Geometry: final body of the model. Coordinates: model frame, mm. A direction names the side the tool comes from. Give positions to 0.01 mm unless a question says otherwise; leave off trailing zeros. Write each loop counter-clockwise with the first axis right and the second up, starting at its lowest first coordinate (ties: lowest second). Pieces come first, ordered by that corner, then holes. Notation, with made-up numbers: (42.25, 59) - (50.25, 59) arc R6 ccw to (50.25, 68) - close; hole circle Ø8 at (48.5, 42.25). An arc over 180 degrees is marked (long way). One line per question, with ' | ' between items. Start each with the question number.
```python
from build123d import *

# Parameters (mm, degrees)
EXTRUDE_2_DEPTH          = 5
FILLET_3_R               = 1
SKETCH_3_R               = 13
SKETCH_3_R_2             = 1.6
CUT_EXTRUDE_5_DEPTH      = 5
CUT_EXTRUDE_6_DEPTH      = 54.322134241
CUT_EXTRUDE_6_DEPTH_BACK = 54.322134241
SKETCH_4_R               = 1.525
CUT_EXTRUDE_7_DEPTH      = 10
FILLET_4_R               = 1.5


with BuildPart() as part:
    # 草圖2 → 填料-伸長2 (new body)
    with BuildSketch(Plane.XY):
        with BuildLine():
            Line((-26.5, 46), (26.5, 46))
            Line((26.5, 46), (26.5, 36))
            Line((26.5, 36), (23, 0))
            ThreePointArc((23, 0), (0, -23), (-23, 0))
            Line((-23, 0), (-26.5, 36))
            Line((-26.5, 36), (-26.5, 46))
        make_face()
    extrude(amount=EXTRUDE_2_DEPTH)

    # 圓角3
    # the kernel refuses this fillet: 1 mm, written as the material it takes off along each edge
    with BuildSketch(Plane(origin=(-26.5, 46, -2.5), x_dir=(0, -1, 0), z_dir=(0, 0, 1)), Plane(origin=(26.5, 46, -2.5), x_dir=(-1, 0, 0), z_dir=(0, 0, 1))) as fillet_3_piece_1:
        with BuildLine():
            CenterArc((FILLET_3_R, FILLET_3_R), FILLET_3_R, 180, 90)
            Line((0, FILLET_3_R), (0, 0))
            Line((0, 0), (FILLET_3_R, 0))
        make_face()
    extrude(amount=10, mode=Mode.SUBTRACT)
    with BuildSketch(Plane(origin=(26.5, 36, -0.121241952), x_dir=(0, 1, 0), z_dir=(0, 0, 1)), Plane(origin=(-26.5, 36, -0.121241952), x_dir=(0.0967659740606196, -0.9953071617667079, 0), z_dir=(0, 0, 1))) as fillet_3_piece_2:
        with BuildLine():
            CenterArc((FILLET_3_R * 0.0484967808039, FILLET_3_R), FILLET_3_R, 264.447028967, 5.552971033)
            Line((-FILLET_3_R * 0.0482691932568, FILLET_3_R * 0.0046928382333), (0, 0))
            Line((0, 0), (FILLET_3_R * 0.0484967808039, 0))
        make_face()
    extrude(amount=5.242483904, mode=Mode.SUBTRACT)

    # 草圖3 → 除料-伸長5 (cut)
    with BuildSketch(Plane.XY):
        Circle(SKETCH_3_R)
        with Locations((18.009998301, 0)):
            Circle(SKETCH_3_R_2)
        with Locations((0, -18.009998301)):
            Circle(SKETCH_3_R_2)
        with Locations((-18.009998301, 0)):
            Circle(SKETCH_3_R_2)
        with Locations((0, 18.009998301)):
            Circle(SKETCH_3_R_2)
        with Locations((11.999602077, 11.999602077)):
            Circle(SKETCH_3_R_2)
        with Locations((11.999602077, -11.999602077)):
            Circle(SKETCH_3_R_2)
        with Locations((-11.999602077, -11.999602077)):
            Circle(SKETCH_3_R_2)
        with Locations((-11.999602077, 11.999602077)):
            Circle(SKETCH_3_R_2)
    extrude(amount=CUT_EXTRUDE_5_DEPTH, mode=Mode.SUBTRACT)

    # 草圖4 → 除料-伸長6 (cut, two sides: drawn at the far end of the back side and taken through both)
    with BuildSketch(Plane.XY.offset(-CUT_EXTRUDE_6_DEPTH_BACK)):
        with Locations((21, 41)):
            Circle(SKETCH_4_R)
        with Locations((7, 41)):
            Circle(SKETCH_4_R)
        with Locations((-7, 41)):
            Circle(SKETCH_4_R)
        with Locations((-21, 41)):
            Circle(SKETCH_4_R)
    extrude(amount=CUT_EXTRUDE_6_DEPTH + CUT_EXTRUDE_6_DEPTH_BACK, mode=Mode.SUBTRACT)

    # 草圖5 → 除料-伸長7 (cut)
    with BuildSketch(Plane.XY.offset(5)):
        Polygon((-21.5, 35), (-6.5, 35), (-20.2, 21), align=None)
        Polygon((11.3, 22.7), (-11.3, 22.7), (0, 34.95), align=None)
        Polygon((6.5, 35), (20.2, 21), (21.5, 35), align=None)
    extrude(amount=-CUT_EXTRUDE_7_DEPTH, mode=Mode.SUBTRACT)

    # 圓角4
    fillet_4_edges = [part.edges().sort_by_distance(p)[0] for p in [
        (6.5, 35, 2.5),
        (21.5, 35, 2.5),
        (20.2, 21, 2.5),
        (-11.3, 22.7, 2.5),
        (0, 34.95, 2.5),
        (11.3, 22.7, 2.5),
        (-20.2, 21, 2.5),
        (-21.5, 35, 2.5),
        (-6.5, 35, 2.5),
    ]]
    fillet(fillet_4_edges, radius=FILLET_4_R)


solid = part.part
```
1) Line query: L1, parallel to Y at x = 7, z = 4 (1 decimal); L2, parallel to Y at x = -5, z = 1.05; L3, parallel to Y at x = -10, z = 2.7. Output: solid intervals per line, ascending.
2) Section C-C, the plane y = -2.5. Output: boundary loops of the cut face in (x, z).
3) Section D-D, the plane x = -7. Output: boundary loops of the cut face in (y, z) (1 decimal), plus the area to 3 significant figures.
4) Section A-A, the plane y = 41. Output: boundary loops of the cut face in (x, z) (3 decimals), plus the area to 3 significant figures.
5) Section B-B, the plane x = 0. Output: boundary loops of the cut face in (y, z), plus the area to 3 significant figures.
6) Reachability of faces 1 (the cylindrical face through (9.26, 23.62, 2.46)), 2 (the flat face through (0, 20, 0)) from +Z, -Z, +X, -X, +Y, -Y: full face, straight path, thin tool, end or side. Return the list, or none.
7) Pull-direction query (X, two-part tool) for faces 3 (the flat face through (-15, 35, 3)), 4 (the cylindrical face through (20.951, 34.523, 2.465)), 5 (the flat face through (0, 20, 5)), 6 (the flat face through (24.772, 18.228, 2.465)); classes: +X half, -X half, draft (parallel to the pull), parting line (faces both ways), or undercut.
8) First-contact query: pin 1 Ø1.8 at (x, y) = (-21, 41) entering from -Z; pin 2 Ø1.5 at (y, z) = (2, 2.5) entering from -X; pin 3 Ø1 at (y, z) = (16.5, 3) entering from +X; pin 4 Ø1.5 at (x, z) = (-15, 2) entering from -Y. Flat tips, straight axial feed; report the tip coordinate or a pass-through.
Answer key:
1) L1: -21.9 to -11, 11 to 22.7, 27.4 to 39.5, 42.5 to 46 | L2: -22.45 to -12, 12 to 22.7, 29.53 to 46 | L3: -20.71 to -8.31, 8.31 to 31.42, 35 to 46
2) outline: (-22.86, 0) - (-12.76, 0) - (-12.76, 5) - (-22.86, 5) - close; (12.76, 0) - (22.86, 0) - (22.86, 5) - (12.76, 5) - close
3) outline: (-21.9, 0) - (-11, 0) - (-11, 5) - (-21.9, 5) - close; (11, 0) - (22.7, 0) - (22.7, 5) - (11, 5) - close; (27.4, 0) - (39.5, 0) - (39.5, 5) - (27.4, 5) - close; (42.5, 0) - (46, 0) - (46, 5) - (42.5, 5) - close | area: 191 mm^2
4) outline: (-26.5, 0) - (-22.525, 0) - (-22.525, 5) - (-26.5, 5) - close; (-19.475, 0) - (-8.525, 0) - (-8.525, 5) - (-19.475, 5) - close; (-5.475, 0) - (5.475, 0) - (5.475, 5) - (-5.475, 5) - close; (8.525, 0) - (19.475, 0) - (19.475, 5) - (8.525, 5) - close; (22.525, 0) - (26.5, 0) - (26.5, 5) - (22.525, 5) - close | area: 204 mm^2
5) outline: (-23, 0) - (-19.61, 0) - (-19.61, 5) - (-23, 5) - close; (-16.41, 0) - (-13, 0) - (-13, 5) - (-16.41, 5) - close; (13, 0) - (16.41, 0) - (16.41, 5) - (13, 5) - close; (19.61, 0) - (22.7, 0) - (22.7, 5) - (19.61, 5) - close; (34.24, 0) - (46, 0) - (46, 5) - (34.24, 5) - close | area: 125 mm^2
6) face 1: +Z, -Z | face 2: -Z, +X, -X, +Y, -Y
7) face 3: undercut | face 4: undercut | face 5: draft | face 6: +X half
8) pin 1: through | pin 2: x = -23.27 | pin 3: x = 24.65 | pin 4: y = -18.05
